CAD build for the part. Positions are in the model's coordinates, mm. Give positions to 0.01 mm unless a question says otherwise; leave off trailing zeros. Write each loop counter-clockwise with the first axis right and the second up, starting at its lowest first coordinate (ties: lowest second). Pieces come first, ordered by that corner, then holes. Notation, with made-up numbers: (-8, -27) - (-3, -27) arc R22 cw to (-3, -15) - close; hole circle Ø2 at (44.25, 28). An arc over 180 degrees is marked (long way). Answer as a JSON object with one key per item and string values.
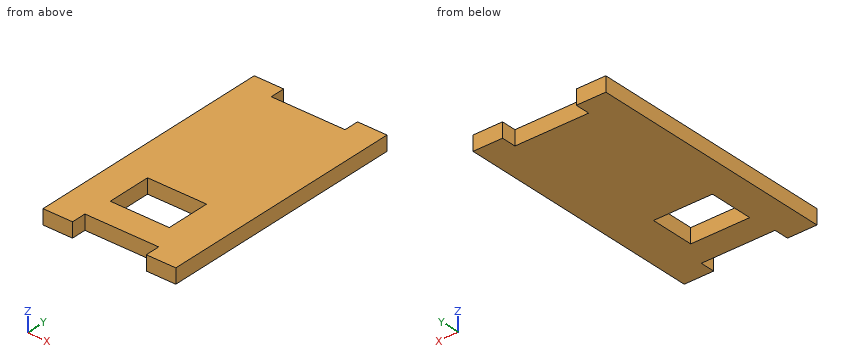
from build123d import *

# Parameters (mm, degrees)
ESQUISSE1_W        = 45
ESQUISSE1_H        = 75
ESQUISSE1_W_2      = 20
ESQUISSE1_H_2      = 15
BOSS_EXTRU_1_DEPTH = 5
ESQUISSE2_W        = 10
ESQUISSE2_H        = 5
BOSS_EXTRU_2_DEPTH = 5


with BuildPart() as part:
    # Esquisse1 → Boss.-Extru.1 (new body)
    with BuildSketch(Plane.XY):
        with Locations((22.5, 37.5)):
            Rectangle(ESQUISSE1_W, ESQUISSE1_H)
        with Locations((21, 16.5)):
            Rectangle(ESQUISSE1_W_2, ESQUISSE1_H_2, mode=Mode.SUBTRACT)
    extrude(amount=BOSS_EXTRU_1_DEPTH)

    # Esquisse2 → Boss.-Extru.2 (add)
    with BuildSketch(Plane.XY.offset(5)):
        with Locations((5, 77.5)):
            Rectangle(ESQUISSE2_W, ESQUISSE2_H)
        with Locations((40, 77.5)):
            Rectangle(ESQUISSE2_W, ESQUISSE2_H)
        with Locations((5, -2.5)):
            Rectangle(ESQUISSE2_W, ESQUISSE2_H)
        with Locations((40, -2.5)):
            Rectangle(ESQUISSE2_W, ESQUISSE2_H)
    extrude(amount=-BOSS_EXTRU_2_DEPTH)


solid = part.part
(1) Flat gauge pin, fed straight in: P1, Ø1.5, axis at x = 22.5, z = 3, coming from the -Y side. Where does the tip first touch, or does it go through?
Answer key:
{"P1": "stops at y = 0"}
(2) Saw through at B-B, the plane x = 24.5. Give the cut face in (y, z), and give its area (3 significant figures).
Answer key:
{"outline": "(0, 0) - (9, 0) - (9, 5) - (0, 5) - close; (24, 0) - (75, 0) - (75, 5) - (24, 5) - close", "area": "300 mm²"}
(3) Probe L1, parallel to Y at x = 14.5, z = 4.35; L2, parallel to X at y = 21, z = 2.2; L3, parallel to X at y = 75.5, z = 1.5. List the from-to ranges inside material, lowest first. Write a range as [from, to].
Answer key:
{"L1": "y = [0, 9], [24, 75]", "L2": "x = [0, 11], [31, 45]", "L3": "x = [0, 10], [35, 45]"}
(4) Saw through at C-C, the plane z = 3.7. Give the cut face in (x, y), and give its area (4 significant figures).
Answer key:
{"outline": "(0, -5) - (10, -5) - (10, 0) - (35, 0) - (35, -5) - (45, -5) - (45, 80) - (35, 80) - (35, 75) - (10, 75) - (10, 80) - (0, 80) - close; hole (11, 9) - (31, 9) - (31, 24) - (11, 24) - close", "area": "3,275 mm²"}
(5) Saw through at A-A, the plane y = 22. Give the cut face in (x, z), and give its area (3 significant figures).
Answer key:
{"outline": "(0, 0) - (11, 0) - (11, 5) - (0, 5) - close; (31, 0) - (45, 0) - (45, 5) - (31, 5) - close", "area": "125 mm²"}
